from build123d import *

# Parameters (mm, degrees)
BOSS_EXTRUDE1_START = -2
BOSS_EXTRUDE1_DEPTH = 2
SKETCH4_R           = 2
CUT_EXTRUDE1_DEPTH  = 2
SKETCH6_R           = 11
CUT_EXTRUDE2_DEPTH  = 1


with BuildPart() as part:
    # Sketch2 → Revolve1 (revolve)
    with BuildSketch(Plane.XY, mode=Mode.PRIVATE) as revolve1_sk:
        Polygon((-10, 3), (-10, 2), (-10, 0), (-15, 0), (-15, 2), (-11, 2), (-11, 3), align=None)
    revolve(revolve1_sk.sketch.rotate(Axis((0, 45.867309825, 0), (0, -1, 0)), 270), axis=Axis((0, 45.867309825, 0), (0, -1, 0)))

    # Sketch3 → Boss-Extrude1 (add)
    with BuildSketch(Plane.XZ.offset(BOSS_EXTRUDE1_START)):
        with BuildLine():
            Line((0, -15), (15, -15))
            ThreePointArc((15, -15), (18.535533906, -13.535533906), (20, -10))
            Line((20, -10), (20, 10))
            ThreePointArc((20, 10), (18.535533906, 13.535533906), (15, 15))
            Line((15, 15), (0, 15))
            ThreePointArc((0, 15), (15, 0), (0, -15))
        make_face()
    extrude(amount=BOSS_EXTRUDE1_DEPTH)

    # Sketch4 → Cut-Extrude1 (cut)
    with BuildSketch(Plane.XZ):
        with Locations(Location((15, 10, 0), (0, 0, 270))):
            Circle(SKETCH4_R)
        with Locations(Location((15, -10, 0), (0, 0, 270))):
            Circle(SKETCH4_R)
    extrude(amount=-CUT_EXTRUDE1_DEPTH, mode=Mode.SUBTRACT)

    # Sketch6 → Cut-Extrude2 (cut)
    with BuildSketch(Plane(origin=(0, 3, 0), x_dir=(1, 0, 0), z_dir=(0, 1, 0))):
        Circle(SKETCH6_R)
    extrude(amount=-CUT_EXTRUDE2_DEPTH, mode=Mode.SUBTRACT)


solid = part.part
Could you check a few things on this model? Use its own coordinates, in mm. Give positions to 0.01 mm unless a question says otherwise; leave off trailing zeros. Write each loop counter-clockwise with the first axis right and the second up, starting at its lowest first coordinate (ties: lowest second). Pieces come first, ordered by that corner, then holes. Notation, with made-up numbers: (14, 30.5) -> (58, 30.5) arc R25 cw to (58, 49.5) -> close; hole circle Ø9 at (29.25, -29.75). An arc over 180 degrees is marked (long way). Answer as CSV lines item,"result". Start each with the question number.
(1) If we section it at B-B, the plane z = 0: Write out the boundary of the cut face in (x, y), and give its area (3 significant figures).
(2) Please list where these lines run through material, in increasing order: line 1 (X direction, y = 1.45, z = 0); line 2 (X direction, y = 1.6, z = 1); line 3 (Z direction, x = -7.5, y = 1.9).
(3) If we section it at C-C, the plane y = 1.7: Write out the boundary of the cut face in (x, z).
(4) I'm going to push flat-ended pins straight in: pin 1 Ø1 at (x, y) = (-8, 1.5) entering from -Z; pin 2 Ø16 at (x, z) = (0, 0) entering from +Y. Where does each tip first touch, or does it pass through?
(5) If we section it at A-A, the plane x = 6: Write out the boundary of the cut face in (y, z), and give its area (3 significant figures).
(6) If we section it at D-D, the plane x = 14: Write out the boundary of the cut face in (y, z), and give its area (3 significant figures).
(7) If we mould it in two halves opening along X, with no side actions, what happens to faces 1 (the face through (-15, 1, 0)), 2 (the face through (19, 1, 13)), 3 (the face through (9.76, 1.01, -2.17))? For each: +X half, -X half, draft (parallel to the pull), parting line (faces both ways), or undercut.
Answer list:
1,outline,"(-15, 0) -> (-10, 0) -> (-10, 2) -> (-15, 2) -> close; (10, 0) -> (20, 0) -> (20, 2) -> (10, 2) -> close"
1,area,"30.0 mm^2"
2,line 1,"-15 to -10, 10 to 20"
2,line 2,"-14.97 to -9.95, 9.95 to 20"
2,line 3,"-12.99 to -6.61, 6.61 to 12.99"
3,outline,"(0, -15) -> (15, -15) arc R5 ccw to (20, -10) -> (20, 10) arc R5 ccw to (15, 15) -> (0, 15) arc R15 ccw to start; hole circle Ø20 at (0, 0); hole circle Ø4 at (15, -10); hole circle Ø4 at (15, 10)"
4,pin 1,"z = -12.99"
4,pin 2,"through"
5,outline,"(0, -15) -> (2, -15) -> (2, -8) -> (0, -8) -> close; (0, 8) -> (2, 8) -> (2, 15) -> (0, 15) -> close"
5,area,"28.0 mm^2"
6,outline,"(0, -15) -> (2, -15) -> (2, -11.73) -> (0, -11.73) -> close; (0, -8.27) -> (2, -8.27) -> (2, 8.27) -> (0, 8.27) -> close; (0, 11.73) -> (2, 11.73) -> (2, 15) -> (0, 15) -> close"
6,area,"46.1 mm^2"
7,face 1,"-X half"
7,face 2,"+X half"
7,face 3,"undercut"
